CAD build for the part. Positions are in the model's coordinates, mm. A direction names the side the tool comes from. Round coordinates to 2 decimals unless told otherwise and drop trailing zeros. Write each loop counter-clockwise with the first axis right and the second up, starting at its lowest first coordinate (ties: lowest second). Pieces come first, ordered by that corner, then holes. Notation, with made-up numbers: (43.25, -36) -> (71.25, -36) arc R25 cw to (71.25, -9) -> close; hole circle Ø8 at (-3.75, 86.25). An arc over 180 degrees is marked (long way). Put each result on its own line as item: value. Start each with the question number.
1. Saw through at C-C on z = 1.5. List the corners of the cut face in (x, y) (3 decimals).
2. Flat gauge pins, fed straight in: P1, Ø1.2, axis at x = -13, z = 3, coming from the +Y side; P2, Ø2.5, axis at y = 13.5, z = 5.5, coming from the +X side; P3, Ø3, axis at y = 15.185, z = 3.965, coming from the -X side; P4, Ø4, axis at y = 16, z = 4, coming from the -X side. Where does each tip first touch, or does it go through?
3. Pull direction Y, two halves, no side cores. Call faces 1 (the flat face through (0, 0, 3)), 2 (the flat face through (-15.06, 8, 3)), 3 (the flat face through (13, 11, 3)), 4 (the cylindrical face through (8.894, 6.699, 2.697)): pulls with the +Y half, pulls with the -Y half, needs draft (parallel to the pull), parting line crosses it, or undercut.
4. Saw through at D-D on y = 8.75. List the corners of the cut face in (x, z), and give its area (3 significant figures).
5. Drill centre lines: line 1 (Y direction, x = -10, z = 3) (3 decimals); line 2 (Y direction, x = 10, z = 3.5) (3 decimals); line 3 (X direction, y = 11.25, z = 2.5). Where is each one in solid material? Low to high. Write a range as from..to.
6. 3-axis set-ups, long thin cutter, end or side, ignore diameter. For faces 5 (the flat face through (10.91, 15, 2)), 6 (the flat face through (-10.91, 15, 2)), 7 (the flat face through (0, 6, 5.32)), 8 (the flat face through (0, 8, 0)), 9 (the cylindrical face through (-13.85, 1.28, 2.62)): which of +Z, -Z, +X, -X, +Y, -Y reach the whole face in a straight line?
7. Saw through at A-A on x = 10. State how many separate pieces and enclosed holes the cut face has, and give its area (3 significant figures).
from build123d import *

# Parameters (mm, degrees)
F1_DEPTH = 5.32
F3_DEPTH = 21.82
F4_DEPTH = 25.971
F5_R     = 1.5
F6_DEPTH = 5.321


with BuildPart() as f1:
    # F0 (on Top) → F1 (new body)
    with BuildSketch(Plane.XY):
        with BuildLine():
            Line((-10.81, 0), (0, 0))
            Line((0, 0), (10.81, 0))
            ThreePointArc((10.81, 0), (13.81520382, 1.24479618), (15.06, 4.25))
            Line((15.06, 4.25), (15.06, 11))
            Line((15.06, 11), (10.91, 11))
            Line((10.91, 11), (10.91, 15.145))
            Line((10.91, 15.145), (-10.91, 15.145))
            Line((-10.91, 15.145), (-10.91, 11))
            Line((-10.91, 11), (-15.06, 11))
            Line((-15.06, 11), (-15.06, 4.25))
            ThreePointArc((-15.06, 4.25), (-13.81520382, 1.24479618), (-10.81, 0))
        make_face()
    extrude(amount=F1_DEPTH)

    # F2 (on face) → F3 (join, through all)
    with BuildSketch(Plane(origin=(-10.91, 0, 0), x_dir=(0, -1, 0), z_dir=(-1, 0, 0))):
        with BuildLine():
            Line((-14.2880050167, 5.32), (-11.4587149867, 5.32))
            ThreePointArc((-11.4587149867, 5.32), (-18.4440319116, 6.2233037881), (-15.145, 0.0002017706))
            Line((-15.145, 0.0002017706), (-15.145, 2.3404923823))
            ThreePointArc((-15.145, 2.3404923823), (-16.7466838062, 4.4141866976), (-14.2880050167, 5.32))
        make_face()
        with BuildLine():
            Line((-15.145, 5.32), (-14.2880050167, 5.32))
            ThreePointArc((-14.2880050167, 5.32), (-16.7466838062, 4.4141866976), (-15.145, 2.3404923823))
            Line((-15.145, 2.3404923823), (-15.145, 5.32))
        make_face()
    extrude(amount=-F3_DEPTH)

    # F2 (on face) → F4 (cut, through all)
    with BuildSketch(Plane(origin=(-10.91, 0, 0), x_dir=(0, -1, 0), z_dir=(-1, 0, 0))):
        with BuildLine():
            Line((-15.145, 5.32), (-14.2880050167, 5.32))
            ThreePointArc((-14.2880050167, 5.32), (-16.7466838062, 4.4141866976), (-15.145, 2.3404923823))
            Line((-15.145, 2.3404923823), (-15.145, 5.32))
        make_face()
        with BuildLine():
            ThreePointArc((-13.56, 3.965), (-13.7535249133, 4.7340930217), (-14.2880050167, 5.32))
            Line((-14.2880050167, 5.32), (-15.145, 5.32))
            Line((-15.145, 5.32), (-15.145, 2.3404923823))
            ThreePointArc((-15.145, 2.3404923823), (-14.0218953186, 2.8301817326), (-13.56, 3.965))
        make_face()
    extrude(amount=-F4_DEPTH, mode=Mode.SUBTRACT)

    # F5 (on face) → F6 (cut, through all)
    with BuildSketch(Plane.XY.offset(5.32)):
        with Locations((-10, 5.685)):
            Circle(F5_R)
        with Locations((10, 5.685)):
            Circle(F5_R)
    extrude(amount=-F6_DEPTH, mode=Mode.SUBTRACT)


solid = f1.part
Return value:
1. outline: (-15.06, 4.25) arc R4.25 ccw to (-10.81, 0) -> (10.81, 0) arc R4.25 ccw to (15.06, 4.25) -> (15.06, 11) -> (10.91, 11) -> (10.91, 18.291) -> (-10.91, 18.291) -> (-10.91, 11) -> (-15.06, 11) -> close; hole circle Ø3 at (-10, 5.685); hole circle Ø3 at (10, 5.685)
2. P1: stops at y = 11
2. P2: stops at x = 10.91
2. P3: passes through
2. P4: stops at x = -10.91
3. face 1: pulls with the -Y half
3. face 2: needs draft
3. face 3: pulls with the +Y half
3. face 4: undercut
4. outline: (-15.06, 0) -> (15.06, 0) -> (15.06, 5.32) -> (-15.06, 5.32) -> close
4. area: 160 mm^2
5. line 1: y = 0..4.185, 7.185..13.878, 16.492..19.031
5. line 2: y = 0..4.185, 7.185..13.628, 16.742..19.123
5. line 3: x = -10.91..10.91
6. face 5: +Z, -Z, +X, +Y
6. face 6: +Z, -Z, -X, +Y
6. face 7: +Z, +X, -X, -Y
6. face 8: -Z, +X, -X, +Y, -Y
6. face 9: +Z, -Z, -X, -Y
7. separate pieces: 2
7. enclosed holes: 1
7. area: 88.3 mm^2
